Print and shaded views of the part. All mm, measured from the part's lowest x, y and z. A direction names the side the tool comes from. Give positions to 0.01 mm unless a question says otherwise; leave off trailing zeros. Write each loop counter-clockwise with the first axis right and the second up, starting at its lowest first coordinate (ties: lowest second). Pieces come first, ordered by that corner, then holes.
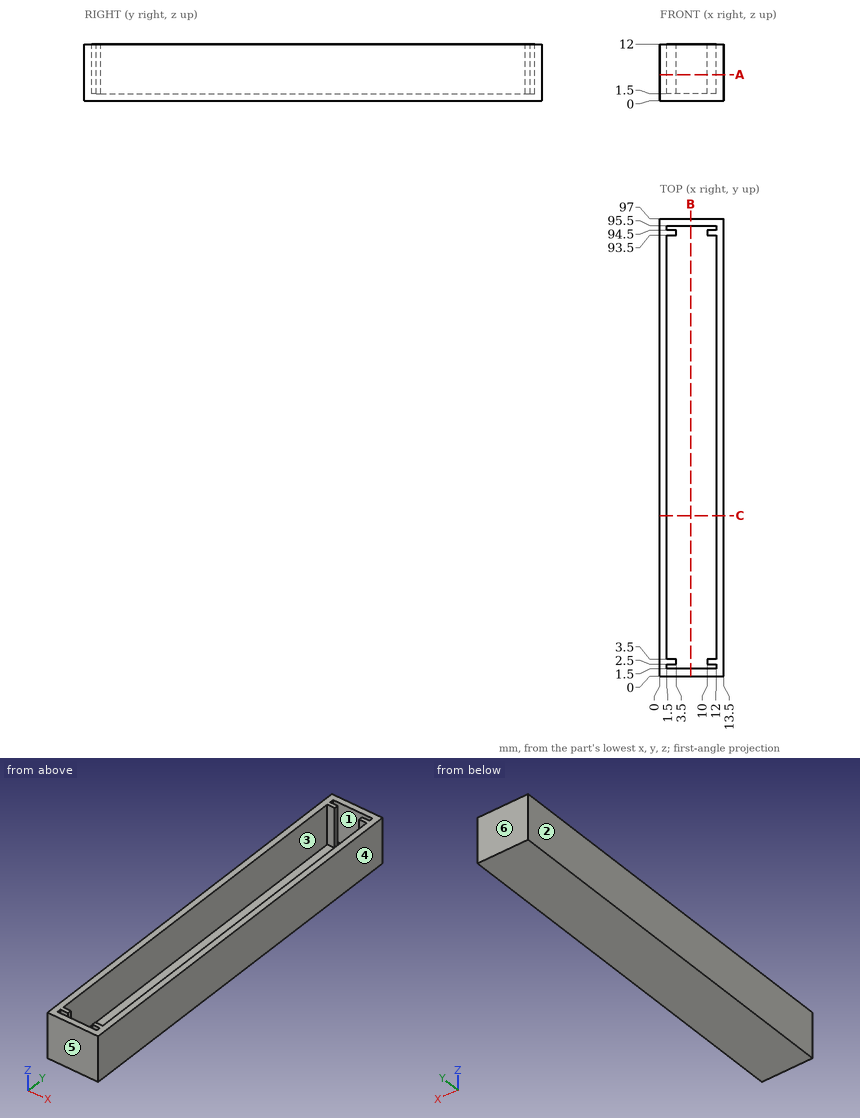
1. Mould opens along Y. For the marked faces 3, 4, 5 and 6 say: pulls with the +Y half, pulls with the -Y half, needs draft (parallel to the pull), parting line crosses it, or undercut.
2. 3-axis set-ups, long thin cutter, end or side, ignore diameter. For the marked faces 1 and 2: which of +Z, -Z, +X, -X, +Y, -Y reach the whole face in a straight line?
3. Drop a flat-ended pin along its axis: pin 1 (3 mm diameter, centred on x = 7.5, y = 56, fed in from +Z). Give the stop position or say it passes through.
4. Saw through at B-B on x = 6.5. Give the cut face in (y, z).
5. Saw through at A-A on z = 5.5. Give the cut face in (x, y), plus the area to 4 significant figures.
6. Saw through at C-C on y = 34. Give the cut face in (x, z).
7. Drill centre lines: line 1 along Y through (x, z) = (10.25, 3.5); line 2 along X through (y, z) = (51, 9.75); line 3 along Y through (x, z) = (5.25, 5). Where is each one in solid material? Low to high.
Outcome:
1. face 3: undercut
1. face 4: needs draft
1. face 5: pulls with the -Y half
1. face 6: pulls with the +Y half
2. face 1: +Z
2. face 2: +Z, -Z, -X, +Y, -Y
3. pin 1: stops at z = 1.5
4. outline: (0, 0) - (97, 0) - (97, 12) - (95.5, 12) - (95.5, 1.5) - (1.5, 1.5) - (1.5, 12) - (0, 12) - close
5. outline: (0, 0) - (13.5, 0) - (13.5, 97) - (0, 97) - close; hole (1.5, 1.5) - (12, 1.5) - (12, 2.5) - (10, 2.5) - (10, 3.5) - (12, 3.5) - (12, 93.5) - (10, 93.5) - (10, 94.5) - (12, 94.5) - (12, 95.5) - (1.5, 95.5) - (1.5, 94.5) - (3.5, 94.5) - (3.5, 93.5) - (1.5, 93.5) - (1.5, 3.5) - (3.5, 3.5) - (3.5, 2.5) - (1.5, 2.5) - close
5. area: 330.5 mm2
6. outline: (0, 0) - (13.5, 0) - (13.5, 12) - (12, 12) - (12, 1.5) - (1.5, 1.5) - (1.5, 12) - (0, 12) - close
7. line 1: y = 0 to 1.5, 2.5 to 3.5, 93.5 to 94.5, 95.5 to 97
7. line 2: x = 0 to 1.5, 12 to 13.5
7. line 3: y = 0 to 1.5, 95.5 to 97
